Geometry check sheet. Reference: the model listing, model coordinates, mm. Round coordinates to 2 decimals unless told otherwise and drop trailing zeros. Write each loop counter-clockwise with the first axis right and the second up, starting at its lowest first coordinate (ties: lowest second). Pieces come first, ordered by that corner, then holes. Notation, with made-up numbers: (67.25, 19) -> (101.25, 19) arc R12 ccw to (101.25, 36) -> close; hole circle Ø6 at (37.25, 5). An arc over 180 degrees is marked (long way). Put each result on its own line as item: value. Start each with the question number.
Autodesk Inventor part; units mm, degrees
ref_plane "Arbeitsebene1" through (-10, 0, 0) normal (0, 0, -1) x (-1, 0, 0)
ref_plane "YZ Plane" through (0, 0, 0) normal (1, 0, 0) x (0, 1, 0)
ref_plane "XZ Plane" through (0, 0, 0) normal (0, 1, 0) x (-1, 0, 0)
sketch "Skizze1" plane through (0, 0, 0) normal (0, 1, 0) x (-1, 0, 0)
  line L0 (0, 10.7628) -> (10, 41)
  line L1 (10, 41) -> (59, 41)
  line L2 (59, 41) -> (69, 10.7628)
  line L3 (69, 10.7628) -> (69, -10.7628)
  line L4 (69, -10.7628) -> (59, -41)
  line L5 (59, -41) -> (10, -41)
  line L6 (10, -41) -> (0, -10.7628)
  line L7 (0, -10.7628) -> (0, 10.7628)
  line L8 (34.5, 41) -> (34.5, -41) construction
  line L9 (0, 0) -> (92.3843, 0) construction
  dimension "d0" = 69
  dimension "d1" = 18.3
  dimension "d2" = 49
  dimension "d4" = 82
  dimension "d5" = 18.3
  dimension "d6" = 18.3
  dimension "d7" = 18.3
extrude "Extrusion1" add sketch "Skizze1" along normal blind 4
sketch "Skizze2" plane through (0, 4, 0) normal (0, 1, 0) x (1, 0, 0)
  line L0 (-69, -10.7628) -> (-59, -41)
  line L1 (-65.2836, -22) -> (-3.7164, -22)
  line L2 (-59, -41) -> (-10, -41)
  line L3 (-59, 41) -> (-69, 10.7628)
  line L4 (-65.2836, 22) -> (-3.7164, 22)
  line L5 (0, 10.7628) -> (-10, 41)
  line L6 (0, 0) -> (-69, 0) construction
  line L7 (-69, 10.7628) -> (-69, -10.7628)
  line L8 (0, -10.7628) -> (0, 10.7628)
  line L9 (-10, -41) -> (0, -10.7628)
  dimension "d10" = 44
extrude "Extrusion2" add sketch "Skizze2" along normal blind 2 contours L7 L3 L4 L5 L8 L9 L1 L0
sketch "Skizze3" plane through (0, 6, 0) normal (0, 1, 0) x (1, 0, 0)
  circle A0 centre (-34.5, 0) radius 22
  line L0 (0, -10.7628) -> (0, 10.7628)
  line L1 (-59, -41) -> (-10, -41)
  point P0 (0, 0)
  point P1 (0, 0)
  point P2 (-34.5, -41)
  dimension "d13" = 44
extrude "Extrusion3" cut sketch "Skizze3" against normal up to surface (6 mm away)
sketch "Skizze4" plane through (0, 4, 0) normal (0, 1, 0) x (1, 0, 0)
  line L0 (-10, 41) -> (-59, 41)
  line L1 (0, 0) -> (-69, 0) construction
  line L2 (-69, 10.7628) -> (-69, -10.7628)
  point P0 (-34.5, 27.5)
  point P1 (-34.5, -27.5)
  point P2 (-34.5, 41)
  dimension "d16" = 55
hole "Bohrung1" at (-34.5, 4, -27.5) at (-34.5, 4, 27.5) direction (0, -1, 0) diameter 4.917 end through all
sketch "Skizze5" plane through (0, 4, 0) normal (0, 1, 0) x (1, 0, 0)
  line L0 (-10, 41) -> (-59, 41)
  line L1 (-34.5, 41) -> (-34.5, 22) construction
  line L2 (0, 0) -> (-76.2503, 0) construction
  point P0 (-17, 31.5)
  point P1 (-52, 31.5)
  point P2 (-34.5, 31.5)
  point P3 (-17, -31.5)
  point P4 (-52, -31.5)
  dimension "d31" = 35
  dimension "d42" = 35
  dimension "d43" = 63
hole "Bohrung2" at (-17, 4, -31.5) at (-52, 4, -31.5) at (-17, 4, 31.5) at (-52, 4, 31.5) direction (0, -1, 0) diameter 6.5 end through all
sketch "Skizze6" plane through (0, 6, 0) normal (0, 1, 0) x (1, 0, 0)
  line L0 (0, -10.7628) -> (0, 10.7628)
  line L1 (-10, 41) -> (-59, 41)
  line L2 (-34.5, 41) -> (-34.5, -41) construction
  line L3 (-59, -41) -> (-10, -41)
  point P0 (0, 0)
  point P1 (-7, 0)
  point P2 (-62, 0)
  point P3 (0, 0)
  point P4 (0, 0)
  dimension "d33" = 55
hole "Bohrung3" at (-7, 6, 0) at (-62, 6, 0) direction (0, -1, 0) diameter 4.134 end through all
ref_plane "Arbeitsebene1" through (-10, 0, 0) normal (0, 0, -1) x (-1, 0, 0)
equation "\"d5\" = d1"
equation "\"d6\" = d1"
equation "\"d7\" = d6"
properties part number "HAlteplatte" material "Stahl, galvanisiert"
(1) Sectioned sample at C-C (y = 2.2). State how many separate pieces and enclosed holes the cut face has, and give its area (3 significant figures).
(2) Go/stop test with flat-tipped pins: pin 1 Ø7.5 at (x, z) = (-52, 31.5) entering from +Y; pin 2 Ø4.5 at (x, z) = (-34.5, -27.5) entering from -Y; pin 3 Ø0.6 at (x, y) = (-43.5, 5.5) entering from -Z; pin 4 Ø0.6 at (x, y) = (-26, 5.5) entering from +Z. Record where each tip stops, or that it passes through.
(3) Sectioned sample at B-B (x = -62). Record the cut outline in (y, z).
(4) Material ranges on L1, parallel to X at y = 3.7, z = 0; L2, parallel to X at y = 1.3, z = 31.5, recorded low to high. Write a range as from..to.
(5) Sectioned sample at A-A (z = 0). Record the cut outline in (x, y), and give its area (3 significant figures).
(6) Mould release check, pull along Z, two halves, no side actions. Record for faces 1 (the cylindrical face through (-17.98, 1.97, -28.4)), 2 (the flat face through (-34, 4, 32)), 3 (the flat face through (-4.93, 2.29, 25.67)): +Z half, -Z half, draft (parallel to the pull), parting line (faces both ways), or undercut.
(7) Sectioned sample at D-D (x = -17). Record the cut outline in (y, z), and give its area (3 significant figures).
Found:
1. separate pieces: 1
1. enclosed holes: 9
1. area: 3,340 mm2
2. pin 1: y = 4
2. pin 2: through
2. pin 3: z = -22
2. pin 4: z = 22
3. outline: (0, -31.93) -> (4, -31.93) -> (4, -22) -> (6, -22) -> (6, -2.07) -> (0, -2.07) -> close; (0, 2.07) -> (6, 2.07) -> (6, 22) -> (4, 22) -> (4, 31.93) -> (0, 31.93) -> close
4. L1: -69..-64.07, -59.93..-56.5, -12.5..-9.07, -4.93..0
4. L2: -62.14..-55.25, -48.75..-20.25, -13.75..-6.86
5. outline: (-69, 0) -> (-64.07, 0) -> (-64.07, 6) -> (-69, 6) -> close; (-59.93, 0) -> (-56.5, 0) -> (-56.5, 6) -> (-59.93, 6) -> close; (-12.5, 0) -> (-9.07, 0) -> (-9.07, 6) -> (-12.5, 6) -> close; (-4.93, 0) -> (0, 0) -> (0, 6) -> (-4.93, 6) -> close
5. area: 100 mm2
6. face 1: undercut
6. face 2: draft
6. face 3: +Z half
7. outline: (0, -41) -> (4, -41) -> (4, -34.75) -> (0, -34.75) -> close; (0, -28.25) -> (4, -28.25) -> (4, -22) -> (6, -22) -> (6, -13.33) -> (0, -13.33) -> close; (0, 13.33) -> (6, 13.33) -> (6, 22) -> (4, 22) -> (4, 28.25) -> (0, 28.25) -> close; (0, 34.75) -> (4, 34.75) -> (4, 41) -> (0, 41) -> close
7. area: 204 mm2
